Check sheet for the modelled part. Datum: model origin and axes. Units: mm. Face numbers are marked on the shaded views. A direction names the side the tool comes from. Coordinates: 2 decimals unless noted, no trailing zeros. Loops run counter-clockwise (first coordinate to the right, second up) from the corner with the lowest first, then second, coordinate; pieces in that order, holes last.
```python
from build123d import *

# Parameters (mm, degrees)
ESQUISSE1_W             = 28
ESQUISSE1_H             = 20
BOSS_EXTRU_1_DEPTH      = 6
ESQUISSE3_W             = 12
ESQUISSE3_H             = 7
ENL_V_MAT_EXTRU_1_DEPTH = 35.928498393
ESQUISSE4_W             = 22
ESQUISSE4_H             = 3
BOSS_EXTRU_2_DEPTH      = 1.5
ESQUISSE5_R             = 0.95
BOSS_EXTRU_3_DEPTH      = 1.9
ESQUISSE6_R             = 0.95
BOSS_EXTRU_4_DEPTH      = 1.9
ESQUISSE12_W            = 28
ESQUISSE12_H            = 5.816034141
BOSS_EXTRU_5_DEPTH      = 20
ESQUISSE13_W            = 8
ESQUISSE13_H            = 14.813855777
BOSS_EXTRU_7_DEPTH      = 20
CHANFREIN4_SIZE         = 14
ESQUISSE15_W            = 10.461102818
ESQUISSE15_H            = 20
BOSS_EXTRU_8_DEPTH      = 20
ESQUISSE16_W            = 10.461102818
ESQUISSE16_H            = 8.2
ENL_V_MAT_EXTRU_2_DEPTH = 20
CONG_3_SIZE             = 6
CONG_4_START            = -29
CONG_4_DEPTH            = 11.461102818
SYM_TRIE3_START         = -8
SYM_TRIE3_DEPTH         = 8
SYM_TRIE3_START_2       = -10.461102818
SYM_TRIE3_2_DEPTH       = 2.461102818


with BuildPart() as part:
    # Esquisse1 → Boss.-Extru.1 (new body)
    with BuildSketch(Plane(origin=(0, 8, 0), x_dir=(1, 0, 0), z_dir=(0, 1, 0))):
        with Locations((-14, -10)):
            Rectangle(ESQUISSE1_W, ESQUISSE1_H)
    extrude(amount=BOSS_EXTRU_1_DEPTH)

    # Esquisse3 → Enlèv. mat.-Extru.1 (cut, through all)
    with BuildSketch(Plane(origin=(0, 14, 0), x_dir=(1, 0, 0), z_dir=(0, 1, 0))):
        with Locations((-14, -10.5)):
            Rectangle(ESQUISSE3_W, ESQUISSE3_H)
    extrude(amount=-ENL_V_MAT_EXTRU_1_DEPTH, mode=Mode.SUBTRACT)

    # Esquisse4 → Boss.-Extru.2 (add)
    with BuildSketch(Plane.XZ.offset(-8)):
        with Locations((-14, 18.5)):
            Rectangle(ESQUISSE4_W, ESQUISSE4_H)
    extrude(amount=BOSS_EXTRU_2_DEPTH)

    # Esquisse5 → Boss.-Extru.3 (add)
    with BuildSketch(Plane.XZ.offset(-8)):
        with Locations(Location((-1.75, 1.75, 0), (0, 0, 90))):
            Circle(ESQUISSE5_R)
    boss_extru_3 = extrude(amount=BOSS_EXTRU_3_DEPTH)

    # Esquisse6 → Boss.-Extru.4 (add)
    with BuildSketch(Plane.XZ.offset(-8)):
        with Locations(Location((-1.5, 17.5, 0), (0, 0, 90))):
            Circle(ESQUISSE6_R)
    boss_extru_4 = extrude(amount=BOSS_EXTRU_4_DEPTH)

    # Symétrie2: Boss.-Extru.3, Boss.-Extru.4 across plane
    add(boss_extru_3.mirror(Plane(origin=(-14, 0, 0), x_dir=(0, 0, 1), z_dir=(1, 0, 0))))
    add(boss_extru_4.mirror(Plane(origin=(-14, 0, 0), x_dir=(0, 0, 1), z_dir=(1, 0, 0))))

    # Esquisse12 → Boss.-Extru.5 (add)
    with BuildSketch(Plane(origin=(0, 14, 0), x_dir=(1, 0, 0), z_dir=(0, 1, 0))):
        with Locations((-14, -17.091982929)):
            Rectangle(ESQUISSE12_W, ESQUISSE12_H)
    extrude(amount=BOSS_EXTRU_5_DEPTH)

    # Esquisse13 → Boss.-Extru.7 (add)
    with BuildSketch(Plane(origin=(0, 14, 0), x_dir=(1, 0, 0), z_dir=(0, 1, 0))):
        with Locations((-24, -7.406927889)):
            Rectangle(ESQUISSE13_W, ESQUISSE13_H)
    extrude(amount=BOSS_EXTRU_7_DEPTH)

    # Chanfrein4
    chanfrein4_edges = [part.edges().sort_by_distance(p)[0] for p in [
        (-24, 34, 0),
    ]]
    chamfer(chanfrein4_edges, length=CHANFREIN4_SIZE)

    # Esquisse15 → Boss.-Extru.8 (add)
    with BuildSketch(Plane.XY.offset(20)):
        with Locations((-22.769448591, 24)):
            Rectangle(ESQUISSE15_W, ESQUISSE15_H)
    extrude(amount=BOSS_EXTRU_8_DEPTH)

    # Esquisse16 → Enlèv. mat.-Extru.2 (cut)
    with BuildSketch(Plane.XY.offset(40)):
        with Locations((-22.769448591, 24.5)):
            Rectangle(ESQUISSE16_W, ESQUISSE16_H)
    extrude(amount=-ENL_V_MAT_EXTRU_2_DEPTH, mode=Mode.SUBTRACT)

    # Congé3
    # a fillet whose section is not a circle: 6 mm, written as the material it takes off along each edge
    with BuildSketch(Plane(origin=(-2.538897182, 14, 40), x_dir=(0, 1, 0), z_dir=(-1, 0, 0))) as cong_3_piece_1:
        with BuildLine():
            Bezier((CONG_3_SIZE, 0), (0, 0), (0, CONG_3_SIZE), weights=[1, 0.424264069, 1])
            Line((0, CONG_3_SIZE), (0, 0))
            Line((0, 0), (CONG_3_SIZE, 0))
        make_face()
    extrude(amount=40.461102818, mode=Mode.SUBTRACT)

    # Congé4: read off the stored shape, not the designer's step
    # Congé4 outline → Congé4 (cut)
    with BuildSketch(Plane.YZ.offset(CONG_4_START)):
        with BuildLine():
            add(Edge.make_bspline(
                [(34, 34.030075377), (34, 39.45727958), (28.6, 40)],
                knots=[0, 0, 0, 1, 1, 1], degree=2, weights=[1, 0.444971909, 1]))
            Line((34, 34.030075377), (34, 40))
            Line((34, 40), (28.6, 40))
        make_face()
    extrude(amount=CONG_4_DEPTH, mode=Mode.SUBTRACT)

    # Symétrie3: read off the stored shape, not the designer's step
    # Symétrie3 outline → Symétrie3 (add)
    with BuildSketch(Plane.YZ.offset(SYM_TRIE3_START)):
        Polygon((34, 14), (34, 14.183965859), (14, 14.183965859), (14, 0), (20, 0), align=None)
        with BuildLine():
            Line((28.6, 40), (28.6, 20))
            Line((28.6, 20), (34, 20))
            Line((34, 20), (34, 34.030075377))
            add(Edge.make_bspline(
                [(28.6, 40), (34, 39.45727958), (34, 34.030075377)],
                knots=[0, 0, 0, 1, 1, 1], degree=2, weights=[1, 0.444971909, 1]))
        make_face()
        with BuildLine():
            add(Edge.make_bspline(
                [(14, 34), (14, 40), (20, 40)],
                knots=[0, 0, 0, 1, 1, 1], degree=2, weights=[1, 0.424264069, 1]))
            Line((14, 34), (14, 20))
            Line((14, 20), (20.4, 20))
            Line((20.4, 20), (20.4, 40))
            Line((20.4, 40), (20, 40))
        make_face()
    extrude(amount=SYM_TRIE3_DEPTH)

    # Sym_trie3 2 outline → Sym_trie3 2 (add)
    with BuildSketch(Plane.YZ.offset(SYM_TRIE3_START_2)):
        with BuildLine():
            Line((28.6, 40), (28.6, 20))
            Line((28.6, 20), (34, 20))
            Line((34, 20), (34, 34.030075377))
            add(Edge.make_bspline(
                [(28.6, 40), (34, 39.45727958), (34, 34.030075377)],
                knots=[0, 0, 0, 1, 1, 1], degree=2, weights=[1, 0.444971909, 1]))
        make_face()
        with BuildLine():
            add(Edge.make_bspline(
                [(14, 34), (14, 40), (20, 40)],
                knots=[0, 0, 0, 1, 1, 1], degree=2, weights=[1, 0.424264069, 1]))
            Line((14, 34), (14, 20))
            Line((14, 20), (20.4, 20))
            Line((20.4, 20), (20.4, 40))
            Line((20.4, 40), (20, 40))
        make_face()
    extrude(amount=SYM_TRIE3_2_DEPTH)


solid = part.part
```
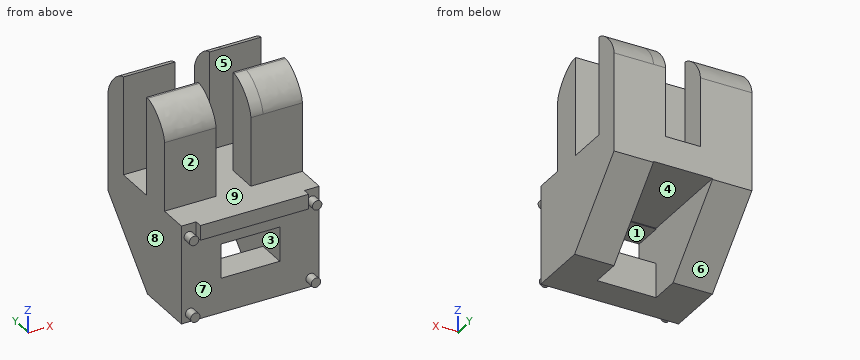
1) Section check C-C on z = 30. Enter the section's corners in (x, y), plus the area to 3 significant figures.
Answer sheet:
outline: (-28, 14) - (-17.54, 14) - (-17.54, 20.4) - (-28, 20.4) - close; (-28, 28.6) - (-17.54, 28.6) - (-17.54, 34) - (-28, 34) - close; (-10.46, 14) - (0, 14) - (0, 20.4) - (-10.46, 20.4) - close; (-10.46, 28.6) - (0, 28.6) - (0, 34) - (-10.46, 34) - close
area: 247 mm2
2) Section check A-A on x = -16.75. Enter the section's corners in (y, z).
Answer sheet:
outline: (6.5, 17) - (8, 17) - (8, 14) - (14, 14) - (14, 14.18) - (34, 14.18) - (34, 20) - (6.5, 20) - close; (8, 0) - (14, 0) - (14, 7) - (8, 7) - close
3) Scan lines: line 1 (X direction, y = 27, z = 7.5); line 2 (Z direction, x = -12, y = 8.25); line 3 (X direction, y = 30, z = 24.5). Record each from-to range of solid material in increasing order.
Answer sheet:
line 1: x = -28 to -20, -8 to 0
line 2: z = 0 to 7, 14 to 20
line 3: x = -28 to -17.54, -10.46 to 0
4) Section check B-B on z = 8.5. Enter the section's corners in (x, y).
Answer sheet:
outline: (-28, 8) - (-20, 8) - (-20, 28.5) - (-28, 28.5) - close; (-8, 8) - (0, 8) - (0, 28.5) - (-8, 28.5) - close
5) Mould release check, pull along Y, two halves, no side actions. Record for the marked faces 6, 7, 8 and 9: +Y half, -Y half, draft (parallel to the pull), parting line (faces both ways), or undercut.
Answer sheet:
face 6: +Y half
face 7: -Y half
face 8: draft
face 9: undercut
6) Section check D-D on y = 9.75. Enter the section's corners in (x, z), plus the area to 3 significant figures.
Answer sheet:
outline: (-28, 0) - (0, 0) - (0, 20) - (-28, 20) - close; hole (-20, 7) - (-8, 7) - (-8, 14) - (-20, 14) - close
area: 476 mm2
7) Set-up check for the marked faces 1, 2, 3, 4 and 5: record each of +Z, -Z, +X, -X, +Y, -Y from which the full face is reachable in a straight line by a thin tool's end or side.
Answer sheet:
face 1: +Y, -Y
face 2: +Z, +X, -X, -Y
face 3: +Y
face 4: -Z, +Y
face 5: +Z, +X, -X
8) Depth check by flat-ended pin: pin 1 (11.5 mm diameter, centred on x = -5.5, z = 29, fed in from -Y); pin 2 (1 mm diameter, centred on x = -9, y = 17.5, fed in from -Z); pin 3 (6 mm diameter, centred on x = -12.5, y = 14, fed in from +Z). Enter the tip coordinate at first touch or a pass-through.
Answer sheet:
pin 1: stops at y = 14
pin 2: stops at z = 14.18
pin 3: stops at z = 37.99
